from build123d import *

# Parameters (mm, degrees)
SALIENTE_EXTRUIR1_DEPTH = 15
CROQUIS2_R              = 2.5
CORTAR_EXTRUIR1_DEPTH   = 20
CROQUIS3_R              = 2.5
CORTAR_EXTRUIR2_DEPTH   = 15


with BuildPart() as part:
    # Croquis1 → Saliente-Extruir1 (new body)
    with BuildSketch(Plane(origin=(0, 0, 0), x_dir=(1, 0, 0), z_dir=(0, 1, 0))):
        with BuildLine():
            Line((0, 0), (23, 0))
            ThreePointArc((23, 0), (24.414213562, 0.585786438), (25, 2))
            Line((25, 2), (25, 25))
            Line((25, 25), (22, 25))
            Line((22, 25), (22, 5))
            ThreePointArc((22, 5), (21.414213562, 3.585786438), (20, 3))
            Line((20, 3), (0, 3))
            Line((0, 3), (0, 0))
        make_face()
    extrude(amount=SALIENTE_EXTRUIR1_DEPTH)

    # Croquis2 → Cortar-Extruir1 (cut)
    with BuildSketch(Plane(origin=(0, 0, -3), x_dir=(-1, 0, 0), z_dir=(0, 0, -1))):
        with Locations((-16, 7.5)):
            Circle(CROQUIS2_R)
        with Locations((-6, 7.5)):
            Circle(CROQUIS2_R)
    extrude(amount=-CORTAR_EXTRUIR1_DEPTH, mode=Mode.SUBTRACT)

    # Croquis3 → Cortar-Extruir2 (cut)
    with BuildSketch(Plane.ZY.offset(-22)):
        with Locations((-9, 7.5)):
            Circle(CROQUIS3_R)
        with Locations((-19, 7.5)):
            Circle(CROQUIS3_R)
    extrude(amount=-CORTAR_EXTRUIR2_DEPTH, mode=Mode.SUBTRACT)


solid = part.part
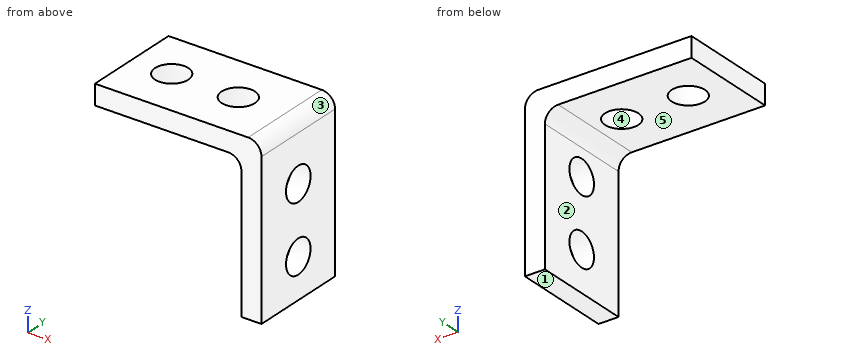
Can you work these out from the model? Positions are in its coordinate system, mm. Face numbers are marked on the shaded views. A direction names the side the tool comes from. Give positions to 0.01 mm unless a question says otherwise; leave off trailing zeros. Loops run counter-clockwise (first coordinate to the right, second up) from the corner with the lowest first, then second, coordinate; pieces in that order, holes last. Notation, with made-up numbers: (-7, 84) - (4, 84) arc R15 cw to (4, 111) - close; hole circle Ø2 at (76, 3.25). An arc over 180 degrees is marked (long way). One line per item, written item: value.
(1) If we section it at C-C, the plane y = 6: List the corners of the cut face in (x, z) for me.
Verdict:
outline: (0, -3) - (4, -3) - (4, 0) - (0, 0) - close; (8, -3) - (14, -3) - (14, 0) - (8, 0) - close; (18, -3) - (20, -3) arc R2 cw to (22, -5) - (22, -7) - (25, -7) - (25, -2) arc R2 ccw to (23, 0) - (18, 0) - close; (22, -25) - (25, -25) - (25, -21) - (22, -21) - close; (22, -17) - (25, -17) - (25, -11) - (22, -11) - close
(2) If we section it at D-D, the plane y = 10.75: List the corners of the cut face in (x, z) for me, plus the area to 3 significant figures.
Verdict:
outline: (0, -3) - (20, -3) arc R2 cw to (22, -5) - (22, -25) - (25, -25) - (25, -2) arc R2 ccw to (23, 0) - (0, 0) - close
area: 141 mm^2
(3) If we section it at A-A, the plane x = 6: List the corners of the cut face in (y, z) for me.
Verdict:
outline: (0, -3) - (5, -3) - (5, 0) - (0, 0) - close; (10, -3) - (15, -3) - (15, 0) - (10, 0) - close
(4) I need wall thicknesses on line 1 along Y through (x, z) = (6, -1); line 2 along Z through (x, y) = (10.25, 9.5); line 3 along X through (y, z) = (10.25, -22). Which ranges of each line are inside material? Lowest first, please.
Verdict:
line 1: 0 to 5, 10 to 15
line 2: -3 to 0
line 3: 22 to 25
(5) If we section it at B-B, the plane z = -19: List the corners of the cut face in (x, y) for me.
Verdict:
outline: (22, 0) - (25, 0) - (25, 5) - (22, 5) - close; (22, 10) - (25, 10) - (25, 15) - (22, 15) - close
(6) On a 3-axis mill with a long thin cutter (end or side, diameter ignored), from which of +Z, -Z, +X, -X, +Y, -Y can I reach the whole of each face in a straight line? I mean the marked faces 1 and 2. Say none if no direction works.
Verdict:
face 1: -Z, +X, -X, +Y, -Y
face 2: -Z, -X, +Y, -Y
(7) If we mould it in two halves opening along X, with no side actions, what happens to the marked faces 3, 4 and 5? For each: released by +X, released by -X, zero draft, split by the parting line, or undercut.
Verdict:
face 3: released by +X
face 4: undercut
face 5: zero draft
(8) I'm going to push flat-ended pins straight in: pin 1 (3 mm diameter, centred on x = 7.5, y = 10.5, fed in from -Z); pin 2 (12 mm diameter, centred on x = 17.5, z = -8.5, fed in from -Y); pin 3 (6 mm diameter, centred on y = 13.5, z = -9.5, fed in from -X). Where does each tip first touch, or does it pass through?
Verdict:
pin 1: z = -3
pin 2: y = 0
pin 3: x = 22
